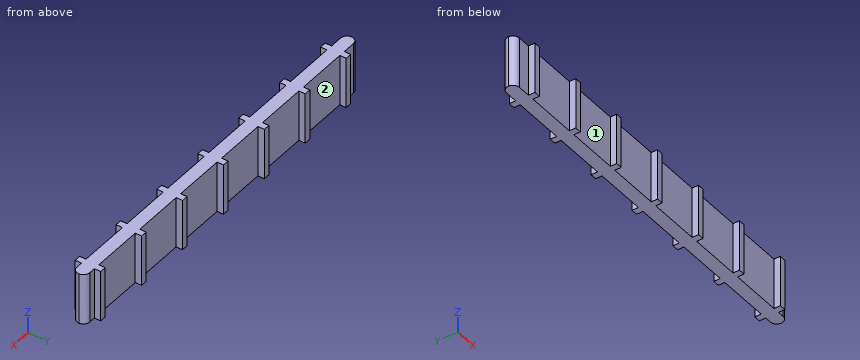
```python
from build123d import *

# Parameters (mm, degrees)
SKETCH1_W           = 300
SKETCH1_H           = 40
BOSS_EXTRUDE1_DEPTH = 10
CUT_EXTRUDE1_DEPTH  = 40
CUT_EXTRUDE2_DEPTH  = 40
SKETCH5_W           = 5
SKETCH5_H           = 40
SKETCH5_W_2         = 2.5
BOSS_EXTRUDE3_DEPTH = 5


with BuildPart() as part:
    # Sketch1 → Boss-Extrude1 (new body)
    with BuildSketch(Plane(origin=(0, 0, 0), x_dir=(1, 0, 0), z_dir=(0, 1, 0))):
        with Locations((-150, 20)):
            Rectangle(SKETCH1_W, SKETCH1_H)
    extrude(amount=BOSS_EXTRUDE1_DEPTH)

    # Sketch2 → Cut-Extrude1 (cut)
    with BuildSketch(Plane(origin=(0, 0, -40), x_dir=(-1, 0, 0), z_dir=(0, 0, -1))):
        with BuildLine():
            Line((0, 10), (0, 5))
            ThreePointArc((0, 5), (1.464466094, 8.535533906), (5, 10))
            Line((5, 10), (0, 10))
        make_face()
        with BuildLine():
            ThreePointArc((5, 0), (1.464466094, 1.464466094), (0, 5))
            Line((0, 5), (0, 0))
            Line((0, 0), (5, 0))
        make_face()
    extrude(amount=-CUT_EXTRUDE1_DEPTH, mode=Mode.SUBTRACT)

    # Sketch4 → Cut-Extrude2 (cut)
    with BuildSketch(Plane(origin=(0, 0, -40), x_dir=(-1, 0, 0), z_dir=(0, 0, -1))):
        with BuildLine():
            Line((300, 10), (295, 10))
            ThreePointArc((295, 10), (298.535533906, 8.535533906), (300, 5))
            Line((300, 5), (300, 10))
        make_face()
        with BuildLine():
            Line((300, 0), (300, 5))
            ThreePointArc((300, 5), (298.535533906, 1.464466094), (295, 0))
            Line((295, 0), (300, 0))
        make_face()
    extrude(amount=-CUT_EXTRUDE2_DEPTH, mode=Mode.SUBTRACT)

    # Sketch5 → Boss-Extrude3 (add)
    with BuildSketch(Plane(origin=(0, 10, 0), x_dir=(1, 0, 0), z_dir=(0, 1, 0))):
        with Locations((-282.5, 20)):
            Rectangle(SKETCH5_W, SKETCH5_H)
        with Locations((-192.5, 20)):
            Rectangle(SKETCH5_W, SKETCH5_H)
        with Locations((-148.75, 20)):
            Rectangle(SKETCH5_W_2, SKETCH5_H)
        with Locations((-146.25, 20)):
            Rectangle(SKETCH5_W_2, SKETCH5_H)
        with Locations((-103.75, 20)):
            Rectangle(SKETCH5_W_2, SKETCH5_H)
        with Locations((-101.25, 20)):
            Rectangle(SKETCH5_W_2, SKETCH5_H)
        with Locations((-58.75, 20)):
            Rectangle(SKETCH5_W_2, SKETCH5_H)
        with Locations((-56.25, 20)):
            Rectangle(SKETCH5_W_2, SKETCH5_H)
        with Locations((-12.5, 20)):
            Rectangle(SKETCH5_W, SKETCH5_H)
        with Locations((-237.5, 20)):
            Rectangle(SKETCH5_W, SKETCH5_H)
    boss_extrude3 = extrude(amount=BOSS_EXTRUDE3_DEPTH)

    # Mirror2: Boss-Extrude3 across plane
    add(boss_extrude3.mirror(Plane.ZX.offset(5)))


solid = part.part
```
Model file for the job. Use its own axes, mm. Face numbers are marked on the shaded views. A direction names the side the tool comes from. Give positions to 0.01 mm unless a question says otherwise; leave off trailing zeros. Order: outer loops, then holes, each group sorted by start corner. A loop starts at its lowest first (then second) coordinate and runs counter-clockwise, first axis right, second up.
1) Saw through at A-A, the plane x = -244.5. Write the cut outline in (y, z), then the cut area to 3 significant figures.
2) Pin check, flat tips, straight feed: pin 1 (1.5 mm diameter, centred on y = -2, z = -23, fed in from +X); pin 2 (1.5 mm diameter, centred on y = 12, z = -28.5, fed in from -X); pin 3 (1 mm diameter, centred on y = 1.5, z = -7.5, fed in from +X). Stop position of each tip, or through.
3) Wall check: probe 1 along X at (y, z) = (4.25, -22.5); probe 2 along Y at (x, z) = (-62, -16); probe 3 along X at (y, z) = (4.75, -24). Give the ranges that are in metal, low to high.
4) 3-axis set-ups, long thin cutter, end or side, ignore diameter. For the marked faces 1 and 2: which of +Z, -Z, +X, -X, +Y, -Y reach the whole face in a straight line?
Computed:
1. outline: (0, -40) - (10, -40) - (10, 0) - (0, 0) - close
1. area: 400 mm2
2. pin 1: stops at x = -10
2. pin 2: stops at x = -285
2. pin 3: stops at x = -1
3. probe 1: x = -299.94 to -0.06
3. probe 2: y = 0 to 10
3. probe 3: x = -299.99 to -0.01
4. face 1: +Z, -Z, -Y
4. face 2: +Z, -Z, +Y
